from build123d import *

# Parameters (mm, degrees)
SKETCH1_W                    = 730
SKETCH1_H                    = 870
SKETCH1_W_2                  = 140
SKETCH1_H_2                  = 723
BASE_FLANGE1_DEPTH           = 0.8
EDGE_FLANGE1_STRIP_W         = 4.8
EDGE_FLANGE1_STRIP_H         = 0.8
EDGE_FLANGE1_STRIP_CUT_DEPTH = 790
EDGE_FLANGE1_DEPTH           = 790


# Sheet-metal steps are written as plain solids
with BuildPart() as part:
    # Sketch1 → Base-Flange1 (new body)
    with BuildSketch(Plane(origin=(0, 0, 0), x_dir=(1, 0, 0), z_dir=(0, 1, 0))):
        Rectangle(SKETCH1_W, SKETCH1_H)
        with Locations((-285, 0)):
            Rectangle(SKETCH1_W_2, SKETCH1_H_2, mode=Mode.SUBTRACT)
    extrude(amount=-BASE_FLANGE1_DEPTH)

    # Edge-Flange1 strip (across the edge) → Edge-Flange1 strip cut (cut)
    with BuildSketch(Plane(origin=(-365, 0, -395), x_dir=(1, 0, 0), z_dir=(0, 0, 1))):
        with Locations((-1.6, -0.4)):
            Rectangle(EDGE_FLANGE1_STRIP_W, EDGE_FLANGE1_STRIP_H)
    extrude(amount=EDGE_FLANGE1_STRIP_CUT_DEPTH, mode=Mode.SUBTRACT)

    # Edge-Flange1 section (across the edge) → Edge-Flange1 (add)
    with BuildSketch(Plane(origin=(-365, 0, -395), x_dir=(1, 0, 0), z_dir=(0, 0, 1))):
        with BuildLine():
            Line((-0.8, 0.8), (-0.8, 40.8))
            Line((-0.8, 40.8), (0, 40.8))
            Line((0, 40.8), (0, 0.8))
            ThreePointArc((0, 0.8), (0.234314575, 0.234314575), (0.8, 0))
            Line((0.8, 0), (0.8, -0.8))
            ThreePointArc((0.8, -0.8), (-0.33137085, -0.33137085), (-0.8, 0.8))
        make_face()
    extrude(amount=EDGE_FLANGE1_DEPTH)


solid = part.part
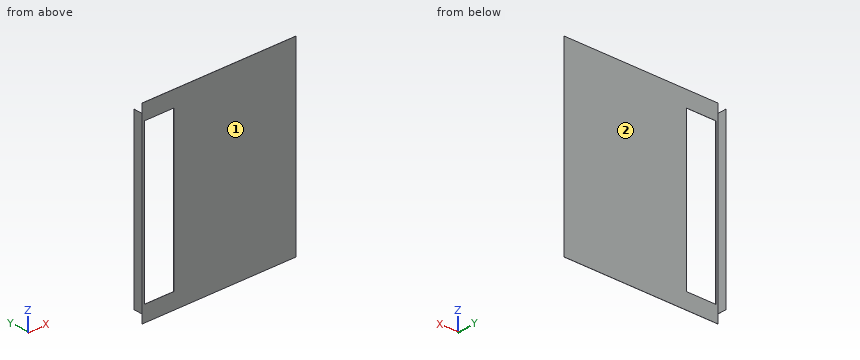
Geometry: final body of the model. Coordinates: model frame, mm. Face numbers are marked on the shaded views. A direction names the side the tool comes from. Give positions to 0.01 mm unless a question says otherwise; leave off trailing zeros. Order: outer loops, then holes, each group sorted by start corner. A loop starts at its lowest first (then second) coordinate and runs counter-clockwise, first axis right, second up. Notation, with made-up numbers: (-6, -23) -> (23, -23) arc R30 ccw to (23, 16) -> close; hole circle Ø3 at (-27.75, 63). An arc over 180 degrees is marked (long way). Put each result on its own line as item: value.
Q1. Section B-B, the plane z = 351. Return loops of the section in (x, y), then the cut area to 3 significant figures.
Here are the results:
outline: (-365.8, 0.8) arc R1.6 ccw to (-364.2, -0.8) -> (-355, -0.8) -> (-355, 0) -> (-364.2, 0) arc R0.8 cw to (-365, 0.8) -> (-365, 40.8) -> (-365.8, 40.8) -> close; (-215, -0.8) -> (365, -0.8) -> (365, 0) -> (-215, 0) -> close
area: 505 mm^2
Q2. Reachability of the marked faces 1 and 2 from +Z, -Z, +X, -X, +Y, -Y: full face, straight path, thin tool, end or side. Return the list, or none.
Here are the results:
face 1: +Z, -Z, +X, -X, -Y
face 2: +Z, -Z, +X, +Y
Q3. Pin query (flat end, axial travel): pin 1 (1 mm diameter, centred on y = 24, z = 67, fed in from +X); pin 2 (0.6 mm diameter, centred on y = -0.5, z = -407.5, fed in from -X); pin 3 (0.6 mm diameter, centred on y = 0, z = -175.5, fed in from -X). Return the tip coordinate at first contact, or that it passes through.
Here are the results:
pin 1: stops at x = -365
pin 2: stops at x = -365
pin 3: stops at x = -365.72
Q4. Section A-A, the plane x = -287.5. Return loops of the section in (y, z).
Here are the results:
outline: (-0.8, -435) -> (0, -435) -> (0, -361.5) -> (-0.8, -361.5) -> close; (-0.8, 361.5) -> (0, 361.5) -> (0, 435) -> (-0.8, 435) -> close
Q5. Section D-D, the plane y = 19. Return loops of the section in (x, z).
Here are the results:
outline: (-365.8, -395) -> (-365, -395) -> (-365, 395) -> (-365.8, 395) -> close
Q6. Material intervals for L1, parallel to X at y = 4.5, z = -242; L2, parallel to Y at x = -87, z = 161.5, sorted ascending.
Here are the results:
L1: x = -365.8 to -365
L2: y = -0.8 to 0
Q7. Section C-C, the plane z = -380. Return loops of the section in (x, y), then the cut area to 3 significant figures.
Here are the results:
outline: (-365.8, 0.8) arc R1.6 ccw to (-364.2, -0.8) -> (365, -0.8) -> (365, 0) -> (-364.2, 0) arc R0.8 cw to (-365, 0.8) -> (-365, 40.8) -> (-365.8, 40.8) -> close
area: 617 mm^2
